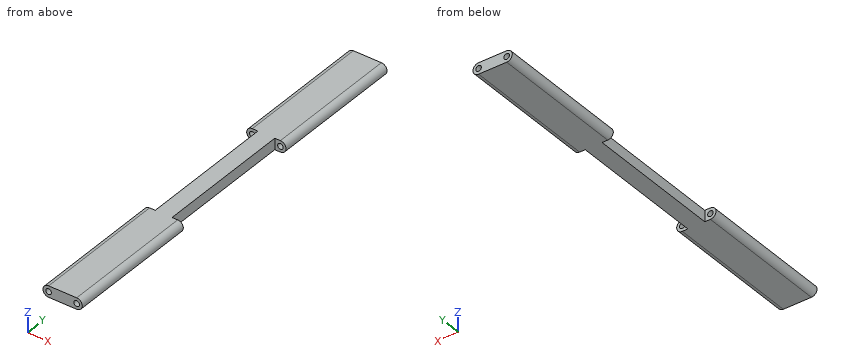
Autodesk Fusion 360 part; units mm, degrees
sketch "Sketch1" plane through (0, 0, 0) normal (0, 1, 0) x (1, 0, 0)
  line L0 (0, 0) -> (10, 0)
  line L1 (10, 0) -> (10, -4)
  line L2 (10, -4) -> (0, -4)
  line L3 (0, -4) -> (0, 0)
  circle A0 centre (0, -2) radius 2
  circle A1 centre (10, -2) radius 2
  circle A2 centre (0, -2) radius 1
  circle A3 centre (10, -2) radius 1
  dimension "d1" = 10
  dimension "d2" = 4
  dimension "d5" = 2
  dimension "d6" = 2
extrude "Extrude1" add sketch "Sketch1" along normal blind 250 contours L3 A0 A2 | L0 L2 A0 A1 | L3 A0 A2 | L1 A1 A3 | L1 A1 A3
ref_plane "WorkPlane1" through (0, 51.2, 0) normal (0, 1, 0) x (0, 0, 1)
sketch "Sketch3" plane through (0, 51.2, 0) normal (0, 1, 0) x (1, 0, 0)
  line L0 (8, -4) -> (8, 0)
  line L1 (10, -4) -> (0, -4)
  line L2 (0, 0) -> (10, 0)
  line L3 (8, -4) -> (10, -4)
  line L4 (8, 0) -> (10, 0)
  circle A0 centre (10, -2) radius 1
  circle A1 centre (10, -2) radius 1
  circle A2 centre (10, -2) radius 2
  arc A3 (10, -4) -> (10, 0) centre (10, -2) ccw
  line L5 (5, 0) -> (5, -4)
  circle A4 centre (0, -2) radius 2
  circle A5 centre (0, -2) radius 1
  line L6 (2, -4) -> (0, -4)
  line L7 (2, -4) -> (2, 0)
  line L8 (2, 0) -> (0, 0)
  dimension "d15" = 2
extrude "Extrude3" cut sketch "Sketch3" against normal blind 49.2 contours L0 L1 L3 A2 | L0 L2 L4 A2 | A2 A3 | L1 A4 L6 L7 | A4 | L2 A4 L7 L8
ref_plane "WorkPlane2" through (0, 125, 0) normal (0, 1, 0) x (0, 0, 1)
mirror "Mirror1" about plane through (0, 125, 0) normal (0, 1, 0) of "Extrude3"
sketch "Sketch4" plane through (0, 125, 0) normal (0, 1, 0) x (1, 0, 0)
  circle A0 centre (10, -2) radius 1
  circle A1 centre (10, -2) radius 2
  circle A2 centre (0, -2) radius 1
  circle A3 centre (0, -2) radius 2
  circle A4 centre (10, -2) radius 1
  arc A5 (10, -4) -> (10, 0) centre (10, -2) ccw
  arc A6 (0, 0) -> (0, -4) centre (0, -2) ccw
  circle A7 centre (0, -2) radius 1
  line L0 (10, -4) -> (0, -4)
  line L1 (0, 0) -> (10, 0)
  line L2 (5, -4) -> (5, 0)
  line L3 (10, 0) -> (8, 0)
  line L4 (8, 0) -> (8, -4)
  line L5 (2, 0) -> (2, -4)
  dimension "d41" = 2
extrude "Extrude8" cut sketch "Sketch4" along normal blind 24.6 and the other way blind 24.6 contours A1 A5 | A1 L1 L3 L4 | A1 L0 L4 | A3 L1 L5 | A3 L0 L5 | A3 A6
extrude "Extrude5" cut 1 faces at (3.6087, 0, 0.4789) along direction (0, 1, 0) blind 52
extrude "Extrude6" cut 1 faces at (3.6087, 250, 0.4789) along direction (0, -1, 0) blind 52
fillet "Fillet2" [suppressed]
equation "d7 = 2 mm + 49.2 mm"
Read the model definition and answer for the solid it produces. Units are mm, in the model's axes. Give positions to 0.01 mm unless a question says otherwise; leave off trailing zeros. Write each loop counter-clockwise with the first axis right and the second up, starting at its lowest first coordinate (ties: lowest second). Pieces come first, ordered by that corner, then holes. Notation, with made-up numbers: (40, 66.5) -> (58, 66.5) arc R24 cw to (58, 103.5) -> close; hole circle Ø4 at (-19.75, -7). An arc over 180 degrees is marked (long way). Answer as a JSON object with one key per item and string values.
1) Section B-B on y = 93 is taken. Write down the section's boundary in (x, z).
Findings below:
{"outline": "(0, 0) -> (10, 0) arc R2 ccw to (10, 4) -> (0, 4) arc R2 ccw to start; hole circle Ø2 at (0, 2); hole circle Ø2 at (10, 2)"}
2) Section A-A on z = 2 is taken. Write down the section's boundary in (x, y), then the cut area to 3 significant figures.
Findings below:
{"outline": "(-2, 52) -> (-1, 52) -> (-1, 100.4) -> (-2, 100.4) -> close; (-2, 149.6) -> (-1, 149.6) -> (-1, 198) -> (-2, 198) -> close; (1, 52) -> (9, 52) -> (9, 100.4) -> (8, 100.4) -> (8, 149.6) -> (9, 149.6) -> (9, 198) -> (1, 198) -> (1, 149.6) -> (2, 149.6) -> (2, 100.4) -> (1, 100.4) -> close; (11, 52) -> (12, 52) -> (12, 100.4) -> (11, 100.4) -> close; (11, 149.6) -> (12, 149.6) -> (12, 198) -> (11, 198) -> close", "area": "1,260 mm^2"}
3) Straight lines are drawn through the part: probe 1 along X at (y, z) = (182.5, 2); probe 2 along Z at (x, y) = (0, 73); probe 3 along Y at (x, z) = (0, 3.55). For each, find the intervals that lie inside material, in ascending order. Write a range as from..to.
Findings below:
{"probe 1": "x = -2..-1, 1..9, 11..12", "probe 2": "z = 0..1, 3..4", "probe 3": "y = 52..100.4, 149.6..198"}
4) Section C-C on y = 139 is taken. Write down the section's boundary in (x, z).
Findings below:
{"outline": "(2, 0) -> (8, 0) -> (8, 4) -> (2, 4) -> close"}
5) A flat-ended cylindrical pin translates along its axis: pin 1 Ø1.2 at (x, z) = (0, 2) entering from +Y. Find the tip coordinate at first contact, or state that the pin passes through.
Findings below:
{"pin 1": "passes through"}
